Work out the finished part from the listing and answer in its coordinate system (mm). Face numbers are marked on the shaded views. A direction names the side the tool comes from. Round coordinates to 2 decimals unless told otherwise and drop trailing zeros. Order: outer loops, then holes, each group sorted by start corner. A loop starts at its lowest first (then second) coordinate and runs counter-clockwise, first axis right, second up. Notation, with made-up numbers: (11, -35) -> (16, -35) arc R31 cw to (16, -11) -> close; hole circle Ø4 at (86, 21). An arc over 180 degrees is marked (long way). Use one line per item in the form item = value.
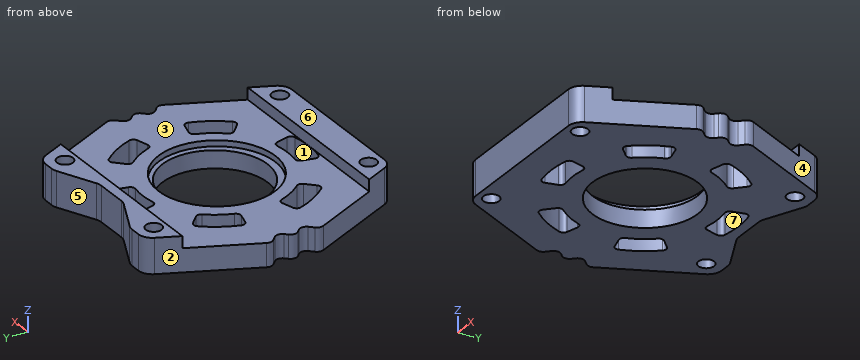
```python
from build123d import *

# Parameters (mm, degrees)
SKETCH1_W           = 69.7357
SKETCH1_H           = 66.8909
SKETCH1_R           = 14.2875
BOSS_EXTRUDE1_DEPTH = 9.525
SKETCH2_W           = 89.996819584
SKETCH2_H           = 50.8
CUT_EXTRUDE1_DEPTH  = 3.175
SKETCH3_R           = 15.875
CUT_EXTRUDE2_DEPTH  = 1.5875
CUT_EXTRUDE3_DEPTH  = 50.245210065
FILLET1_R           = 3.81
FILLET2_R           = 1.778
CUT_EXTRUDE4_DEPTH  = 49.991669707
SKETCH6_R           = 2.159
CUT_EXTRUDE5_DEPTH  = 49.991669707


with BuildPart() as part:
    # Sketch1 → Boss-Extrude1 (new body)
    with BuildSketch(Plane.XY):
        Rectangle(SKETCH1_W, SKETCH1_H)
        with Locations(Location((0, 0, 0), (0, 0, 180))):
            Circle(SKETCH1_R, mode=Mode.SUBTRACT)
    extrude(amount=BOSS_EXTRUDE1_DEPTH)

    # Sketch2 → Cut-Extrude1 (cut)
    with BuildSketch(Plane.XY.offset(9.525)):
        Rectangle(SKETCH2_W, SKETCH2_H)
    extrude(amount=-CUT_EXTRUDE1_DEPTH, mode=Mode.SUBTRACT)

    # Sketch3 → Cut-Extrude2 (cut)
    with BuildSketch(Plane.XY.offset(6.35)):
        with Locations((0, -0.50165)):
            Circle(SKETCH3_R)
    extrude(amount=-CUT_EXTRUDE2_DEPTH, mode=Mode.SUBTRACT)

    # Sketch4 → Cut-Extrude3 (cut, through all)
    with BuildSketch(Plane(origin=(0, 0, 0), x_dir=(-1, 0, 0), z_dir=(0, 0, -1))):
        Polygon((-34.86785, 6.551654679), (-22.346309376, 33.44545), (-34.86785, 33.44545), align=None)
        Polygon((-31.592022661, 3.275827339), (-34.86785, 6.551654679), (-34.86785, 0), align=None)
        Polygon((-31.592022661, -3.275827339), (-34.86785, 0), (-34.86785, -6.551654679), align=None)
        Polygon((-22.346309376, -33.44545), (-34.86785, -6.551654679), (-34.86785, -33.44545), align=None)
        Polygon((34.86785, -33.44545), (34.86785, -6.551654679), (22.346309376, -33.44545), align=None)
        Polygon((-5.118898156, 28.176296472), (5.118898156, 28.176296472), (16.435998884, 33.44545), (-16.435998884, 33.44545), align=None)
        Polygon((34.86785, 33.44545), (22.346309376, 33.44545), (34.86785, 6.551654679), align=None)
        Polygon((34.86785, 0), (34.86785, 6.551654679), (31.592022661, 3.275827339), align=None)
        Polygon((34.86785, -6.551654679), (34.86785, 0), (31.592022661, -3.275827339), align=None)
    extrude(amount=-CUT_EXTRUDE3_DEPTH, mode=Mode.SUBTRACT)

    # Fillet1
    fillet1_edges = [part.edges().sort_by_distance(p)[0] for p in [
        (-5.118898156, 28.176296472, 4.7625),
        (5.118898156, 28.176296472, 4.7625),
        (16.435998884, 33.44545, 4.7625),
        (-16.435998884, 33.44545, 4.7625),
        (-22.346309376, 33.44545, 4.7625),
        (22.346309376, 33.44545, 4.7625),
        (22.346309376, -33.44545, 4.7625),
        (-22.346309376, -33.44545, 4.7625),
    ]]
    fillet(fillet1_edges, radius=FILLET1_R)

    # Fillet2
    fillet2_edges = [part.edges().sort_by_distance(p)[0] for p in [
        (31.592022661, -3.275827339, 3.175),
        (-34.86785, 6.551654679, 3.175),
        (-34.86785, 0, 3.175),
        (-31.592022661, 3.275827339, 3.175),
        (-31.592022661, -3.275827339, 3.175),
        (34.86785, 6.551654679, 3.175),
        (31.592022661, 3.275827339, 3.175),
        (34.86785, 0, 3.175),
        (34.86785, -6.551654679, 3.175),
        (-34.86785, -6.551654679, 3.175),
    ]]
    fillet(fillet2_edges, radius=FILLET2_R)

    # Sketch5 → Cut-Extrude4 (cut, through all)
    with BuildSketch(Plane(origin=(0, 0, 0), x_dir=(-1, 0, 0), z_dir=(0, 0, -1))):
        with BuildLine():
            Line((5.214806052, 20.196856995), (6.024138943, 23.3313898))
            ThreePointArc((6.024138943, 23.3313898), (5.871123899, 24.322469299), (5.046807084, 24.893568211))
            ThreePointArc((5.046807084, 24.893568211), (0, 25.4), (-5.046807084, 24.893568211))
            ThreePointArc((-5.046807084, 24.893568211), (-5.871123899, 24.322469299), (-6.024138943, 23.3313898))
            Line((-6.024138943, 23.3313898), (-5.214806052, 20.196856995))
            ThreePointArc((-5.214806052, 20.196856995), (-4.663096918, 19.440454734), (-3.742950076, 19.267662556))
            ThreePointArc((-3.742950076, 19.267662556), (0, 19.62785), (3.742950076, 19.267662556))
            ThreePointArc((3.742950076, 19.267662556), (4.663096918, 19.440454734), (5.214806052, 20.196856995))
        make_face()
        with BuildLine():
            Line((20.09839426, 5.58227398), (23.217645744, 6.44863754))
            ThreePointArc((23.217645744, 6.44863754), (23.999438245, 7.076692204), (24.081866003, 8.076120962))
            ThreePointArc((24.081866003, 8.076120962), (21.997045256, 12.7), (19.035058919, 16.817447248))
            ThreePointArc((19.035058919, 16.817447248), (18.128314346, 17.245777095), (17.193506801, 16.88275226))
            Line((17.193506801, 16.88275226), (14.883588208, 14.614583014))
            ThreePointArc((14.883588208, 14.614583014), (14.504379202, 13.758587758), (14.814810207, 12.875321128))
            ThreePointArc((14.814810207, 12.875321128), (16.998216722, 9.813925), (18.557760282, 6.392341427))
            ThreePointArc((18.557760282, 6.392341427), (19.16747612, 5.681866976), (20.09839426, 5.58227398))
        make_face()
        with BuildLine():
            Line((14.883588208, -14.614583014), (17.193506801, -16.88275226))
            ThreePointArc((17.193506801, -16.88275226), (18.128314346, -17.245777095), (19.035058919, -16.817447248))
            ThreePointArc((19.035058919, -16.817447248), (21.997045256, -12.7), (24.081866003, -8.076120962))
            ThreePointArc((24.081866003, -8.076120962), (23.999438245, -7.076692204), (23.217645744, -6.44863754))
            Line((23.217645744, -6.44863754), (20.09839426, -5.58227398))
            ThreePointArc((20.09839426, -5.58227398), (19.16747612, -5.681866976), (18.557760282, -6.392341427))
            ThreePointArc((18.557760282, -6.392341427), (16.998216722, -9.813925), (14.814810207, -12.875321128))
            ThreePointArc((14.814810207, -12.875321128), (14.504379202, -13.758587758), (14.883588208, -14.614583014))
        make_face()
        with BuildLine():
            Line((-5.214806052, -20.196856995), (-6.024138943, -23.3313898))
            ThreePointArc((-6.024138943, -23.3313898), (-5.871123899, -24.322469299), (-5.046807084, -24.893568211))
            ThreePointArc((-5.046807084, -24.893568211), (0, -25.4), (5.046807084, -24.893568211))
            ThreePointArc((5.046807084, -24.893568211), (5.871123899, -24.322469299), (6.024138943, -23.3313898))
            Line((6.024138943, -23.3313898), (5.214806052, -20.196856995))
            ThreePointArc((5.214806052, -20.196856995), (4.663096918, -19.440454734), (3.742950076, -19.267662556))
            ThreePointArc((3.742950076, -19.267662556), (0, -19.62785), (-3.742950076, -19.267662556))
            ThreePointArc((-3.742950076, -19.267662556), (-4.663096918, -19.440454734), (-5.214806052, -20.196856995))
        make_face()
        with BuildLine():
            Line((-20.09839426, -5.58227398), (-23.217645744, -6.44863754))
            ThreePointArc((-23.217645744, -6.44863754), (-23.999438245, -7.076692204), (-24.081866003, -8.076120962))
            ThreePointArc((-24.081866003, -8.076120962), (-21.997045256, -12.7), (-19.035058919, -16.817447248))
            ThreePointArc((-19.035058919, -16.817447248), (-18.128314346, -17.245777095), (-17.193506801, -16.88275226))
            Line((-17.193506801, -16.88275226), (-14.883588208, -14.614583014))
            ThreePointArc((-14.883588208, -14.614583014), (-14.504379202, -13.758587758), (-14.814810207, -12.875321128))
            ThreePointArc((-14.814810207, -12.875321128), (-16.998216722, -9.813925), (-18.557760282, -6.392341427))
            ThreePointArc((-18.557760282, -6.392341427), (-19.16747612, -5.681866976), (-20.09839426, -5.58227398))
        make_face()
        with BuildLine():
            Line((-14.883588208, 14.614583014), (-17.193506801, 16.88275226))
            ThreePointArc((-17.193506801, 16.88275226), (-18.128314346, 17.245777095), (-19.035058919, 16.817447248))
            ThreePointArc((-19.035058919, 16.817447248), (-21.997045256, 12.7), (-24.081866003, 8.076120962))
            ThreePointArc((-24.081866003, 8.076120962), (-23.999438245, 7.076692204), (-23.217645744, 6.44863754))
            Line((-23.217645744, 6.44863754), (-20.09839426, 5.58227398))
            ThreePointArc((-20.09839426, 5.58227398), (-19.16747612, 5.681866976), (-18.557760282, 6.392341427))
            ThreePointArc((-18.557760282, 6.392341427), (-16.998216722, 9.813925), (-14.814810207, 12.875321128))
            ThreePointArc((-14.814810207, 12.875321128), (-14.504379202, 13.758587758), (-14.883588208, 14.614583014))
        make_face()
    extrude(amount=-CUT_EXTRUDE4_DEPTH, mode=Mode.SUBTRACT)

    # Sketch6 → Cut-Extrude5 (cut, through all)
    with BuildSketch(Plane.XY.offset(9.525)):
        with Locations((-19.05, 28.70835)):
            Circle(SKETCH6_R)
        with Locations((19.05, 28.70835)):
            Circle(SKETCH6_R)
        with Locations((-19.05, -29.71165)):
            Circle(SKETCH6_R)
        with Locations((19.05, -29.71165)):
            Circle(SKETCH6_R)
    extrude(amount=-CUT_EXTRUDE5_DEPTH, mode=Mode.SUBTRACT)


solid = part.part
```
Item 1: For the marked faces 5, 6 and 7, determine the directions among +Z, -Z, +X, -X, +Y, -Y from which every point of the face is accessible in a straight line to the end or side of a thin tool.
Findings:
face_5 = +Z, -Z, +Y
face_6 = +Z, +X, -X, +Y, -Y
face_7 = +Z, -Z
Item 2: The part is cut by section B-B, the plane x = -2.5. Give the number of separate pieces and of enclosed holes in the cut face, and give its area (3 significant figures).
Findings:
separate_pieces = 4
enclosed_holes = 0
area = 168 mm^2
Item 3: The part is cut by section A-A, the plane z = 8.25. Give the vertices of the cut face in (x, y), and give its area (3 significant figures).
Findings:
outline = (-26.09, -25.4) -> (-23.37, -31.24) arc R3.81 ccw to (-19.92, -33.45) -> (19.92, -33.45) arc R3.81 ccw to (23.37, -31.24) -> (26.09, -25.4) -> close; (-26.09, 25.4) -> (26.09, 25.4) -> (23.37, 31.24) arc R3.81 ccw to (19.92, 33.45) -> (17.28, 33.45) arc R3.81 ccw to (15.67, 33.09) -> (5.88, 28.53) arc R3.81 cw to (4.28, 28.18) -> (-4.28, 28.18) arc R3.81 cw to (-5.88, 28.53) -> (-15.67, 33.09) arc R3.81 ccw to (-17.28, 33.45) -> (-19.92, 33.45) arc R3.81 ccw to (-23.37, 31.24) -> close; hole circle Ø4.32 at (-19.05, -29.71); hole circle Ø4.32 at (-19.05, 28.71); hole circle Ø4.32 at (19.05, -29.71); hole circle Ø4.32 at (19.05, 28.71)
area = 603 mm^2
Item 4: Consider line 1 along X through (y, z) = (11.5, 1.5); line 2 along Y through (x, z) = (19.05, 5.75); line 3 along X through (y, z) = (-10, 5.25). Determine where each line is inside the solid, lowest interval first.
Findings:
line_1 = -32.56 to -22.65, -15.91 to -8.48, 8.48 to 15.91, 22.65 to 32.56
line_2 = -33.45 to -31.87, -27.55 to -16.8, -5.75 to 5.75, 16.8 to 26.55, 30.87 to 33.45
line_3 = -33.26 to -23.35, -16.89 to -12.72, 12.72 to 16.89, 23.35 to 33.26
Item 5: A flat-ended cylindrical pin translates along its axis: P1, Ø3.5, axis at x = -12, z = 8.5, coming from the +Y side. Find the tip coordinate at first contact, or state that the pin passes through.
Findings:
P1 = 32.19
Item 6: Determine the mould class of the marked faces 1, 2, 3 and 4 for opening direction X: released by +X, released by -X, zero draft, split by the parting line, or undercut.
Findings:
face_1 = undercut
face_2 = released by -X
face_3 = zero draft
face_4 = released by +X
